```python
from build123d import *

# Parameters (mm, degrees)
EXTRUDE_1_DEPTH                    = 160
SKETCH_2_W                         = 250
SKETCH_2_H                         = 160
EXTRUDE_2_DEPTH                    = 160
PATTERN_CIRCULAR_1_COUNT           = 3
SKETCH_3_W                         = 633.811978465
SKETCH_3_H                         = 120
CUT_EXTRUDE_1_DEPTH                = 70
SKETCH_4_W                         = 250
SKETCH_4_H                         = 120
CUT_EXTRUDE_2_DEPTH                = 60
SKETCH_5_W                         = 250
SKETCH_5_H                         = 120
CUT_EXTRUDE_3_DEPTH                = 60
SKETCH_6_W                         = 60
SKETCH_6_H                         = 120
EXTRUDE_3_DEPTH                    = 20
PATTERN_CIRCULAR_4_COUNT           = 3
PATTERN_CIRCULAR_4_COPY_1_SKETCH_W = 633.811978465
PATTERN_CIRCULAR_4_COPY_1_SKETCH_H = 120
PATTERN_CIRCULAR_4_COPY_1_DEPTH    = 70
PATTERN_CIRCULAR_4_COPY_2_SKETCH_W = 633.811978465
PATTERN_CIRCULAR_4_COPY_2_SKETCH_H = 120
PATTERN_CIRCULAR_4_COPY_2_DEPTH    = 70
CUT_EXTRUDE_4_DEPTH                = 120
M14X1_5_1_D                        = 12.5
PATTERN_CIRCULAR_5_COUNT           = 3


with BuildPart() as part:
    # 草圖1 → 填料-伸長1 (new body)
    with BuildSketch(Plane(origin=(0, 0, 0), x_dir=(1, 0, 0), z_dir=(0, 1, 0))):
        Polygon((-80, 46.188021535), (-80, 680), (80, 680), (80, 46.188021535), (628.897274573, -270.717967697), (548.897274573, -409.282032303), (0, -92.37604307), (-548.897274573, -409.282032303), (-628.897274573, -270.717967697), align=None)
    extrude(amount=EXTRUDE_1_DEPTH)

    # 草圖2 → 填料-伸長2 (add)
    with BuildSketch(Plane(origin=(0, 160, 0), x_dir=(1, 0, 0), z_dir=(0, 1, 0))):
        with Locations((0, 760)):
            Rectangle(SKETCH_2_W, SKETCH_2_H)
    extrude_2 = extrude(amount=-EXTRUDE_2_DEPTH)

    # 環狀複製排列1: 填料-伸長2 ×3 about axis
    pattern_circular_1_axis = Axis((0, 0, 0), (0, 1, 0))
    for i in range(1, PATTERN_CIRCULAR_1_COUNT):
        add(extrude_2.rotate(pattern_circular_1_axis, i * 360 / PATTERN_CIRCULAR_1_COUNT))

    # 草圖3 → 除料-伸長1 (cut)
    with BuildSketch(Plane(origin=(80, 0, 0), x_dir=(0, 0, -1), z_dir=(1, 0, 0))):
        with Locations((363.094010767, 80)):
            Rectangle(SKETCH_3_W, SKETCH_3_H)
    cut_extrude_1 = extrude(amount=-CUT_EXTRUDE_1_DEPTH, mode=Mode.SUBTRACT)

    # 鏡射1: 除料-伸長1 across plane
    add(cut_extrude_1.mirror(Plane(origin=(0, 0, 0), x_dir=(0, 0, 1), z_dir=(1, 0, 0))), mode=Mode.SUBTRACT)

    # 草圖4 → 除料-伸長2 (cut)
    with BuildSketch(Plane.XY.offset(-680)):
        with Locations((0, 80)):
            Rectangle(SKETCH_4_W, SKETCH_4_H)
    cut_extrude_2 = extrude(amount=-CUT_EXTRUDE_2_DEPTH, mode=Mode.SUBTRACT)

    # 草圖5 → 除料-伸長3 (cut)
    with BuildSketch(Plane(origin=(0, 0, -840), x_dir=(-1, 0, 0), z_dir=(0, 0, -1))):
        with Locations((0, 80)):
            Rectangle(SKETCH_5_W, SKETCH_5_H)
    cut_extrude_3 = extrude(amount=-CUT_EXTRUDE_3_DEPTH, mode=Mode.SUBTRACT)

    # 草圖6 → 填料-伸長3 (add)
    with BuildSketch(Plane.ZY.offset(10)):
        with Locations((-710, 80)):
            Rectangle(SKETCH_6_W, SKETCH_6_H)
    extrude_3 = extrude(amount=-EXTRUDE_3_DEPTH)

    # 環狀複製排列4: 除料-伸長1, 除料-伸長2, 除料-伸長3, 填料-伸長3 ×3 about axis
    pattern_circular_4_axis = Axis((0, 0, 0), (0, 1, 0))
    add([cut_extrude_1.rotate(pattern_circular_4_axis, i * 360 / PATTERN_CIRCULAR_4_COUNT) for i in range(1, PATTERN_CIRCULAR_4_COUNT)], mode=Mode.SUBTRACT)
    add([cut_extrude_2.rotate(pattern_circular_4_axis, i * 360 / PATTERN_CIRCULAR_4_COUNT) for i in range(1, PATTERN_CIRCULAR_4_COUNT)], mode=Mode.SUBTRACT)
    add([cut_extrude_3.rotate(pattern_circular_4_axis, i * 360 / PATTERN_CIRCULAR_4_COUNT) for i in range(1, PATTERN_CIRCULAR_4_COUNT)], mode=Mode.SUBTRACT)
    add([extrude_3.rotate(pattern_circular_4_axis, i * 360 / PATTERN_CIRCULAR_4_COUNT) for i in range(1, PATTERN_CIRCULAR_4_COUNT)])

    # 環狀複製排列4 copy 1 sketch → 環狀複製排列4 copy 1 (cut)
    with BuildSketch(Plane(origin=(40, 0, 69.282032303), x_dir=(-0.8660254037844387, 0, 0.4999999999999998), z_dir=(0.4999999999999998, 0, 0.8660254037844387))):
        with Locations((363.094010767, -80)):
            Rectangle(PATTERN_CIRCULAR_4_COPY_1_SKETCH_W, PATTERN_CIRCULAR_4_COPY_1_SKETCH_H)
    extrude(amount=-PATTERN_CIRCULAR_4_COPY_1_DEPTH, mode=Mode.SUBTRACT)

    # 環狀複製排列4 copy 2 sketch → 環狀複製排列4 copy 2 (cut)
    with BuildSketch(Plane(origin=(40, 0, -69.282032303), x_dir=(0.8660254037844384, 0, 0.5000000000000004), z_dir=(0.5000000000000004, 0, -0.8660254037844384))):
        with Locations((363.094010767, -80)):
            Rectangle(PATTERN_CIRCULAR_4_COPY_2_SKETCH_W, PATTERN_CIRCULAR_4_COPY_2_SKETCH_H)
    extrude(amount=-PATTERN_CIRCULAR_4_COPY_2_DEPTH, mode=Mode.SUBTRACT)

    # 草圖7 → 除料-伸長4 (cut)
    with BuildSketch(Plane(origin=(0, 20, 0), x_dir=(1, 0, 0), z_dir=(0, 1, 0))):
        Polygon((-10, 46.188021535), (-80, 46.188021535), (-45, -14.43375673), (-10, 5.773502692), align=None)
        Polygon((10, 46.188021535), (80, 46.188021535), (45, -14.43375673), (10, 5.773502692), align=None)
        Polygon((-35, -31.754264805), (0, -11.547005384), (35, -31.754264805), (0, -92.37604307), align=None)
    extrude(amount=CUT_EXTRUDE_4_DEPTH, mode=Mode.SUBTRACT)

    # M14x1.5 螺紋孔1 (through all)
    with Locations(Plane(origin=(0, 160, 0), x_dir=(-1, 0, 0), z_dir=(0, 1, 0))):
        with Locations((27, -803), (-27, -803), (-27, -717), (27, -717)):
            m14x1_5_1 = Hole(M14X1_5_1_D / 2)

    # 環狀複製排列5: M14x1.5 螺紋孔1 ×3 about axis
    pattern_circular_5_axis = Axis((0, 0, 0), (0, 1, 0))
    for i in range(1, PATTERN_CIRCULAR_5_COUNT):
        add(m14x1_5_1.rotate(pattern_circular_5_axis, i * 360 / PATTERN_CIRCULAR_5_COUNT), mode=Mode.SUBTRACT)


solid = part.part
```
Check sheet for the modelled part. Datum: model origin and axes. Units: mm. A direction names the side the tool comes from. Give positions to 0.01 mm unless a question says otherwise; leave off trailing zeros. Order: outer loops, then holes, each group sorted by start corner. A loop starts at its lowest first (then second) coordinate and runs counter-clockwise, first axis right, second up. Notation, with made-up numbers: (52.25, 71.5) -> (82.25, 71.5) arc R13 cw to (82.25, 81.5) -> close; hole circle Ø10 at (61, 31.5). An arc over 180 degrees is marked (long way). Use CSV: the item, a comma, the result in double quotes. Start each with the question number.
1) Sectioned sample at B-B, the plane y = 58. Record the boundary of the cut face in (x, z).
2) Sectioned sample at C-C, the plane x = 379.5. Record the boundary of the cut face in (y, z).
3) Mould release check, pull along X, two halves, no side actions. Record for faces 1 (the face through (125, 81, -759)), 2 (the face through (675.01, 80.84, 310.85)), 3 (the face through (-726.586, 10.14, 421.516)): released by +X, released by -X, zero draft, split by the parting line, or undercut.
4) Material ranges on line 1 (X direction, y = 15.5, z = -803); line 2 (Y direction, x = 49.5, z = -242); line 3 (Z direction, x = 27, y = 146), recorded low to high. Write a range as from..to.
5) Set-up check for faces 4 (the face through (-703, 140, 404)), 5 (the face through (2, 140, -810)), 6 (the face through (-175, 140, 17)): record each of +Z, -Z, +X, -X, +Y, -Y from which the full face is reachable in a straight line by a thin tool's end or side.
6) Go/stop test with flat-tipped pins: P1, Ø2, axis at y = 37.5, z = -33.5, coming from the -X side; P2, Ø5, axis at y = 143.5, z = 100.5, coming from the +X side; P3, Ø2, axis at x = 353, y = 21.5, coming from the +Z side. Record where each tip stops, or that it passes through.
7) Sectioned sample at A-A, the plane z = -223.5. Record the boundary of the cut face in (x, y), plus the area to 3 significant figures.
Recorded:
1,outline,"(-738, 281.75) -> (-703.36, 261.75) -> (-645.86, 361.34) -> (-10, -5.77) -> (-10, -740) -> (-125, -740) -> (-125, -780) -> (125, -780) -> (125, -740) -> (10, -740) -> (10, -5.77) -> (645.86, 361.34) -> (703.36, 261.75) -> (738, 281.75) -> (613, 498.25) -> (578.36, 478.25) -> (635.86, 378.66) -> (0, 11.55) -> (-635.86, 378.66) -> (-578.36, 478.25) -> (-613, 498.25) -> close"
2,outline,"(0, 126.73) -> (20, 126.73) -> (20, 207.56) -> (140, 207.56) -> (140, 126.73) -> (160, 126.73) -> (160, 311.48) -> (140, 311.48) -> (140, 230.65) -> (20, 230.65) -> (20, 311.48) -> (0, 311.48) -> close"
3,face 1,"released by +X"
3,face 2,"undercut"
3,face 3,"released by -X"
4,line 1,"-125..-33.25, -20.75..20.75, 33.25..125"
4,line 2,"0..20, 140..160"
4,line 3,"-840..-809.25, -796.75..-723.25, -710.75..107.96"
5,face 4,"+Z, -X"
5,face 5,"-Z, +X, -X"
5,face 6,"none"
6,P1,"x = -10"
6,P2,"x = 338.4"
6,P3,"z = 215.93"
7,outline,"(-80, 0) -> (80, 0) -> (80, 20) -> (10, 20) -> (10, 140) -> (80, 140) -> (80, 160) -> (-80, 160) -> (-80, 140) -> (-10, 140) -> (-10, 20) -> (-80, 20) -> close"
7,area,"8,800 mm2"
